from build123d import *

# Parameters (mm, degrees)
SKETCH1_R           = 9.525
SKETCH1_R_2         = 6.35
BOSS_EXTRUDE1_DEPTH = 152.4
SKETCH2_W           = 3.175
SKETCH2_H           = 25.179063452
CUT_EXTRUDE1_DEPTH  = 10


with BuildPart() as part:
    # Sketch1 → Boss-Extrude1 (new body)
    with BuildSketch(Plane.XY):
        Circle(SKETCH1_R)
        Circle(SKETCH1_R_2, mode=Mode.SUBTRACT)
    extrude(amount=BOSS_EXTRUDE1_DEPTH)

    # Sketch2 → Cut-Extrude1 (cut)
    with BuildSketch(Plane.XY.offset(152.4)):
        Rectangle(SKETCH2_W, SKETCH2_H)
    extrude(amount=-CUT_EXTRUDE1_DEPTH, mode=Mode.SUBTRACT)


solid = part.part
Part model, mm, in its own coordinate system. A direction names the side the tool comes from. Give positions to 0.01 mm unless a question says otherwise; leave off trailing zeros. Write each loop counter-clockwise with the first axis right and the second up, starting at its lowest first coordinate (ties: lowest second). Pieces come first, ordered by that corner, then holes.
1) Which spindle directions (+Z, -Z, +X, -X, +Y, -Y) get a long thin tool onto all of the face, cutting with end or side? Do faces 1 (the face through (-6.5, 0.1, 152.4)), 2 (the face through (0, -8, 142.4)). Say none if no direction does.
Resolved:
face 1: +Z, +X, -X, +Y, -Y
face 2: +Z, +Y, -Y
2) Probe L1, parallel to Y at x = 0.25, z = 113; L2, parallel to Y at x = 1.5, z = 111; L3, parallel to X at y = -1.25, z = 70. List the from-to ranges inside material, lowest first.
Resolved:
L1: y = -9.52 to -6.35, 6.35 to 9.52
L2: y = -9.41 to -6.17, 6.17 to 9.41
L3: x = -9.44 to -6.23, 6.23 to 9.44
3) Cut at B-B on x = 0. Write the cut outline in (y, z) (3 decimals), then the cut area to 3 significant figures.
Resolved:
outline: (-9.525, 0) - (-6.35, 0) - (-6.35, 142.4) - (-9.525, 142.4) - close; (6.35, 0) - (9.525, 0) - (9.525, 142.4) - (6.35, 142.4) - close
area: 904 mm2
4) Cut at A-A on y = 0. Write the cut outline in (x, z) (3 decimals), then the cut area to 3 significant figures.
Resolved:
outline: (-9.525, 0) - (-6.35, 0) - (-6.35, 152.4) - (-9.525, 152.4) - close; (6.35, 0) - (9.525, 0) - (9.525, 152.4) - (6.35, 152.4) - close
area: 968 mm2
5) Cut at C-C on z = 24. Write the cut outline in (x, y) (3 decimals).
Resolved:
outline: circle Ø19.05 at (0, 0); hole circle Ø12.7 at (0, 0)
6) Cut at D-D on x = 8.25. Write the cut outline in (y, z).
Resolved:
outline: (-4.76, 0) - (4.76, 0) - (4.76, 152.4) - (-4.76, 152.4) - close
7) Pin check, flat tips, straight feed: pin 1 (3.5 mm diameter, centred on x = 0.5, y = 7, fed in from +Z); pin 2 (1.5 mm diameter, centred on x = -6.5, z = 50, fed in from -Y); pin 3 (1.6 mm diameter, centred on y = 7, z = 148, fed in from -X); pin 4 (4 mm diameter, centred on y = -3, z = 135.5, fed in from +X). Stop position of each tip, or through.
Resolved:
pin 1: stops at z = 152.4
pin 2: stops at y = -7.59
pin 3: stops at x = -7.23
pin 4: stops at x = 9.47
